The model under review builds one solid part; all positions refer to its coordinate system, in mm. A direction names the side the tool comes from. Round coordinates to 2 decimals unless told otherwise and drop trailing zeros. Write each question's results on one line, items separated by ' | '. Start each with the question number.
Item 1: We need section A-A (y = 448.5). Give the number of separate pieces and of enclosed holes in the cut face, and give its area (3 significant figures).
Item 2: Clearance check with flat-ended pins moving along their axes: pin 1 Ø0.7 at (y, z) = (171, -13.5) entering from -X; pin 2 Ø0.9 at (y, z) = (171.5, -14.5) entering from -X; pin 3 Ø1.5 at (x, z) = (23, 3.5) entering from +Y; pin 4 Ø5 at (x, y) = (-13, 138.5) entering from -Z. State where each tip first meets the part, or that it passes through.
Item 3: Mouldability with a two-part tool opening along X and no side actions: class faces 3 (the flat face through (15, 246, -5.8)), 4 (the flat face through (-30, 246, 9)), 5 (the flat face through (0, 246, -15)) as pulls with the +X half, pulls with the -X half, needs draft (parallel to the pull), parting line crosses it, or undercut.
Item 4: For L1, parallel to X at y = 195.5, z = -0.25; L2, parallel to Z at x = -20, y = 429.5; L3, parallel to X at y = 419.5, z = -9.25, list the stretches that pass through material, from the lowest coordinate up. Write a range as from..to.
Item 5: Tool access review of faces 1 (the flat face through (30, 246, 9)), 2 (the flat face through (9.2, 246, 0)): name each direction out of +Z, -Z, +X, -X, +Y, -Y from which nothing blocks a thin tool from reaching the whole face with its end or side.
from build123d import *

# Parameters (mm, degrees)
F0_W      = 60
F0_H      = 30
F1_DEPTH  = 500
F2_R      = 3.65
F3_DEPTH  = 500.001
F5_DEPTH  = 500.001
F6_R      = 2
F8_DEPTH  = 500.001
F10_DEPTH = 500.001
F11_W     = 0.8
F11_H     = 0.8
F12_DEPTH = 500.001


with BuildPart() as f1:
    # F0 (on Front) → F1 (new body)
    with BuildSketch(Plane.XZ):
        Rectangle(F0_W, F0_H)
    extrude(amount=-F1_DEPTH)

    # F2 (on face) → F3 (cut, through all)
    with BuildSketch(Plane.XZ):
        with Locations((-15, 0)):
            Circle(F2_R)
        with Locations((15, 0)):
            Circle(F2_R)
    extrude(amount=-F3_DEPTH, mode=Mode.SUBTRACT)

    # F4 (on face) → F5 (cut, through all)
    with BuildSketch(Plane.XZ):
        Polygon((-11, 15), (-15, 15), (-19, 15), (-19, 12.8), (-23, 12.8), (-23, 8.8), (-20, 5.8), (-15, 5.8), (-10, 5.8), (-7, 8.8), (-7, 12.8), (-11, 12.8), align=None)
        Polygon((19, 12.8), (19, 15), (15, 15), (11, 15), (11, 12.8), (7, 12.8), (7, 8.8), (10, 5.8), (15, 5.8), (20, 5.8), (23, 8.8), (23, 12.8), align=None)
        Polygon((23.8, 8), (20.8, 5), (20.8, 0), (20.8, -5), (23.8, -8), (27.8, -8), (27.8, -4), (30, -4), (30, 0), (30, 4), (27.8, 4), (27.8, 8), align=None)
        Polygon((23, -8.8), (20, -5.8), (15, -5.8), (10, -5.8), (7, -8.8), (7, -12.8), (11, -12.8), (11, -15), (15, -15), (19, -15), (19, -12.8), (23, -12.8), align=None)
        Polygon((-20.8, 0), (-20.8, 5), (-23.8, 8), (-27.8, 8), (-27.8, 4), (-30, 4), (-30, 0), (-30, -4), (-27.8, -4), (-27.8, -8), (-23.8, -8), (-20.8, -5), align=None)
        Polygon((-23, -12.8), (-19, -12.8), (-19, -15), (-15, -15), (-11, -15), (-11, -12.8), (-7, -12.8), (-7, -8.8), (-10, -5.8), (-15, -5.8), (-20, -5.8), (-23, -8.8), align=None)
        Polygon((-5.3, 8.9), (-9.2, 5), (-9.2, 0), (-9.2, -5), (-5.3, -8.9), (-5.3, -12.8), (0, -12.8), (5.3, -12.8), (5.3, -8.9), (9.2, -5), (9.2, 0), (9.2, 5), (5.3, 8.9), (5.3, 12.8), (0, 12.8), (-5.3, 12.8), align=None)
    extrude(amount=-F5_DEPTH, mode=Mode.SUBTRACT)

    # F6
    f6_edges = [f1.edges().sort_by_distance(p)[0] for p in [
        (-30, 250, 15),
        (30, 250, 15),
        (30, 250, -15),
        (-30, 250, -15),
    ]]
    fillet(f6_edges, radius=F6_R)

    # F7 (on face) → F8 (cut, through all)
    with BuildSketch(Plane.XZ):
        with BuildLine():
            Line((-27.8, 9.5), (-24.5, 9.5))
            Line((-24.5, 9.5), (-24.5, 12.8))
            Line((-24.5, 12.8), (-26.8, 12.8))
            ThreePointArc((-26.8, 12.8), (-27.507107, 12.507107), (-27.8, 11.8))
            Line((-27.8, 11.8), (-27.8, 9.5))
        make_face()
        with BuildLine():
            Line((26.8, 12.8), (24.5, 12.8))
            Line((24.5, 12.8), (24.5, 9.5))
            Line((24.5, 9.5), (27.8, 9.5))
            Line((27.8, 9.5), (27.8, 11.8))
            ThreePointArc((27.8, 11.8), (27.507107, 12.507107), (26.8, 12.8))
        make_face()
        with BuildLine():
            Line((24.5, -12.8), (26.8, -12.8))
            ThreePointArc((26.8, -12.8), (27.507107, -12.507107), (27.8, -11.8))
            Line((27.8, -11.8), (27.8, -9.5))
            Line((27.8, -9.5), (24.5, -9.5))
            Line((24.5, -9.5), (24.5, -12.8))
        make_face()
        with BuildLine():
            Line((-24.5, -9.5), (-27.8, -9.5))
            Line((-27.8, -9.5), (-27.8, -11.8))
            ThreePointArc((-27.8, -11.8), (-27.507107, -12.507107), (-26.8, -12.8))
            Line((-26.8, -12.8), (-24.5, -12.8))
            Line((-24.5, -12.8), (-24.5, -9.5))
        make_face()
    extrude(amount=-F8_DEPTH, mode=Mode.SUBTRACT)

    # F9 (on face) → F10 (cut, through all)
    with BuildSketch(Plane.XZ):
        Polygon((-18.641792, 2.841792), (-17.949755, 2.149755), (-17.216416, 2.9), (-17.9, 3.583584), align=None)
        Polygon((-17.841792, -3.641792), (-17.149755, -2.949755), (-17.9, -2.216416), (-18.583584, -2.9), align=None)
        Polygon((-11.358208, -2.841792), (-12.050245, -2.149755), (-12.783584, -2.9), (-12.1, -3.583584), align=None)
        Polygon((-12.158208, 3.641792), (-12.850245, 2.949755), (-12.1, 2.216416), (-11.416416, 2.9), align=None)
        Polygon((11.416416, 2.9), (12.1, 2.216416), (12.850245, 2.949755), (12.158208, 3.641792), align=None)
        Polygon((17.216416, 2.9), (17.949755, 2.149755), (18.641792, 2.841792), (17.9, 3.583584), align=None)
        Polygon((17.841792, -3.641792), (18.583584, -2.9), (17.9, -2.216416), (17.149755, -2.949755), align=None)
        Polygon((12.783584, -2.9), (12.050245, -2.149755), (11.358208, -2.841792), (12.1, -3.583584), align=None)
    extrude(amount=-F10_DEPTH, mode=Mode.SUBTRACT)

    # F11 (on face) → F12 (cut, through all)
    with BuildSketch(Plane.XZ):
        with Locations((10.6, 14.6)):
            Rectangle(F11_W, F11_H)
        with Locations((19.4, 14.6)):
            Rectangle(F11_W, F11_H)
        with Locations((29.6, -4.4)):
            Rectangle(F11_W, F11_H)
        with Locations((29.6, 4.4)):
            Rectangle(F11_W, F11_H)
        with Locations((10.6, -14.6)):
            Rectangle(F11_W, F11_H)
        with Locations((19.4, -14.6)):
            Rectangle(F11_W, F11_H)
        with Locations((-10.6, 14.6)):
            Rectangle(F11_W, F11_H)
        with Locations((-19.4, 14.6)):
            Rectangle(F11_W, F11_H)
        with Locations((-29.6, 4.4)):
            Rectangle(F11_W, F11_H)
        with Locations((-29.6, -4.4)):
            Rectangle(F11_W, F11_H)
        with Locations((-19.4, -14.6)):
            Rectangle(F11_W, F11_H)
        with Locations((-10.6, -14.6)):
            Rectangle(F11_W, F11_H)
    extrude(amount=-F12_DEPTH, mode=Mode.SUBTRACT)


solid = f1.part
Here are the results:
1) separate pieces: 1 | enclosed holes: 7 | area: 551 mm2
2) pin 1: stops at x = -29.99 | pin 2: stops at x = -29.7 | pin 3: passes through | pin 4: stops at z = -14.2
3) face 3: undercut | face 4: pulls with the -X half | face 5: needs draft
4) L1: x = -20.8..-18.64, -11.36..-9.2, 9.2..11.36, 18.64..20.8 | L2: z = -15..-12.8, -5.8..5.8, 12.8..15 | L3: x = -30..-23, -7..-5.3, 5.3..7, 23..30
5) face 1: +Z, -Z, +X, +Y, -Y | face 2: +Y, -Y
